The listing builds one solid part. Answer for the finished solid, in the listing's coordinates (mm). Face numbers are marked on the shaded views. A direction names the side the tool comes from. Coordinates: 2 decimals unless noted, no trailing zeros. Loops run counter-clockwise (first coordinate to the right, second up) from the corner with the lowest first, then second, coordinate; pieces in that order, holes last. Notation, with made-up numbers: M 77,50.5 L 87,50.5 A8 cw 87,63.5 Z; hole C 56.5,29.25 d8. An arc over 180 degrees is marked long. Answer as a JSON object with one key per item and string values. Group by question number.
1. A cutting plane is placed at A-A on y = 0. Give the vertices of the cut face in (x, z).
2. A cutting plane is placed at D-D on y = -23. Give the vertices of the cut face in (x, z).
3. Straight lines are drawn through the part: L1, parallel to Y at x = 0, z = 1.05; L2, parallel to Y at x = 0, z = 6.25; L3, parallel to Z at x = 4.5, y = 26.5. For each, find the intervals that lie inside material, in ascending order.
4. Given pin 1 (1.5 mm diameter, centred on x = 5, z = 5, fed in from -Y); pin 2 (1 mm diameter, centred on y = -16, z = 6, fed in from -X); pin 3 (1.5 mm diameter, centred on x = 17, z = 3.5, fed in from -Y), each flat-ended and moving along its own axis, determine where each tip first touches the part or whether it passes through.
5. Determine the mould class of the marked faces 4, 5 and 6 for opening direction X: released by +X, released by -X, zero draft, split by the parting line, or undercut.
6. For the marked faces 1, 2 and 3, determine the directions among +Z, -Z, +X, -X, +Y, -Y from which every point of the face is accessible in a straight line to the end or side of a thin tool.
7. A cutting plane is placed at C-C on z = 4.5. Give the vertices of the cut face in (x, y), and give its area (3 significant figures).
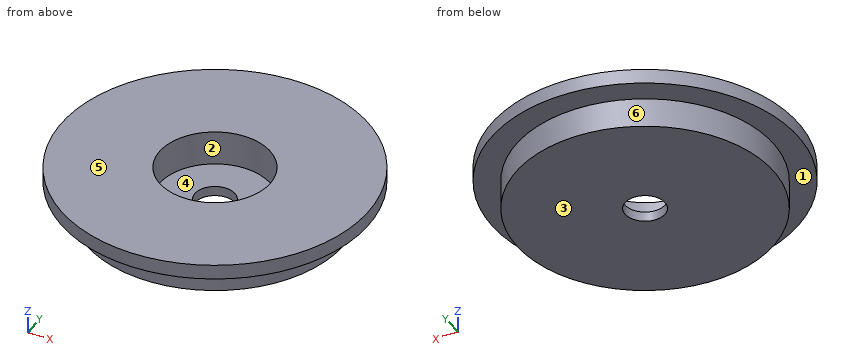
from build123d import *

# Parameters (mm, degrees)
SKETCH_R     = 26
SKETCH_R_2   = 4.05
PAD_DEPTH    = 6
SKETCH001_R  = 31
PAD001_DEPTH = 3
SKETCH002_R  = 11.2
POCKET_DEPTH = 7


with BuildPart() as part:
    # Sketch → Pad (new body)
    with BuildSketch(Plane.XY):
        Circle(SKETCH_R)
        Circle(SKETCH_R_2, mode=Mode.SUBTRACT)
    extrude(amount=PAD_DEPTH)

    # Sketch001 (on Face4 of Pad) → Pad001 (join)
    with BuildSketch(Plane.XY.offset(6)):
        Circle(SKETCH001_R)
    extrude(amount=PAD001_DEPTH)

    # Sketch002 (on Face3 of Pad001) → Pocket (cut)
    with BuildSketch(Plane.XY.offset(9)):
        Circle(SKETCH002_R)
    extrude(amount=-POCKET_DEPTH, mode=Mode.SUBTRACT)


solid = part.part
From the geometry:
{
 "1": {"outline": "M -31,6 L -26,6 L -26,0 L -4.05,0 L -4.05,2 L -11.2,2 L -11.2,9 L -31,9 Z; M 4.05,0 L 26,0 L 26,6 L 31,6 L 31,9 L 11.2,9 L 11.2,2 L 4.05,2 Z"},
 "2": {"outline": "M -20.78,6 L -12.12,6 L -12.12,0 L 12.12,0 L 12.12,6 L 20.78,6 L 20.78,9 L -20.78,9 Z"},
 "3": {"L1": "y = -26 to -4.05, 4.05 to 26", "L2": "y = -31 to -11.2, 11.2 to 31", "L3": "z = 6 to 9"},
 "4": {"pin 1": "stops at y = -25.65", "pin 2": "stops at x = -26.85", "pin 3": "stops at y = -20.3"},
 "5": {"face 4": "undercut", "face 5": "zero draft", "face 6": "split by the parting line"},
 "6": {"face 1": "-Z", "face 2": "+Z", "face 3": "-Z, +X, -X, +Y, -Y"},
 "7": {"outline": "C 0,0 d52; hole C 0,0 d22.4", "area": "1,730 mm²"}
}
